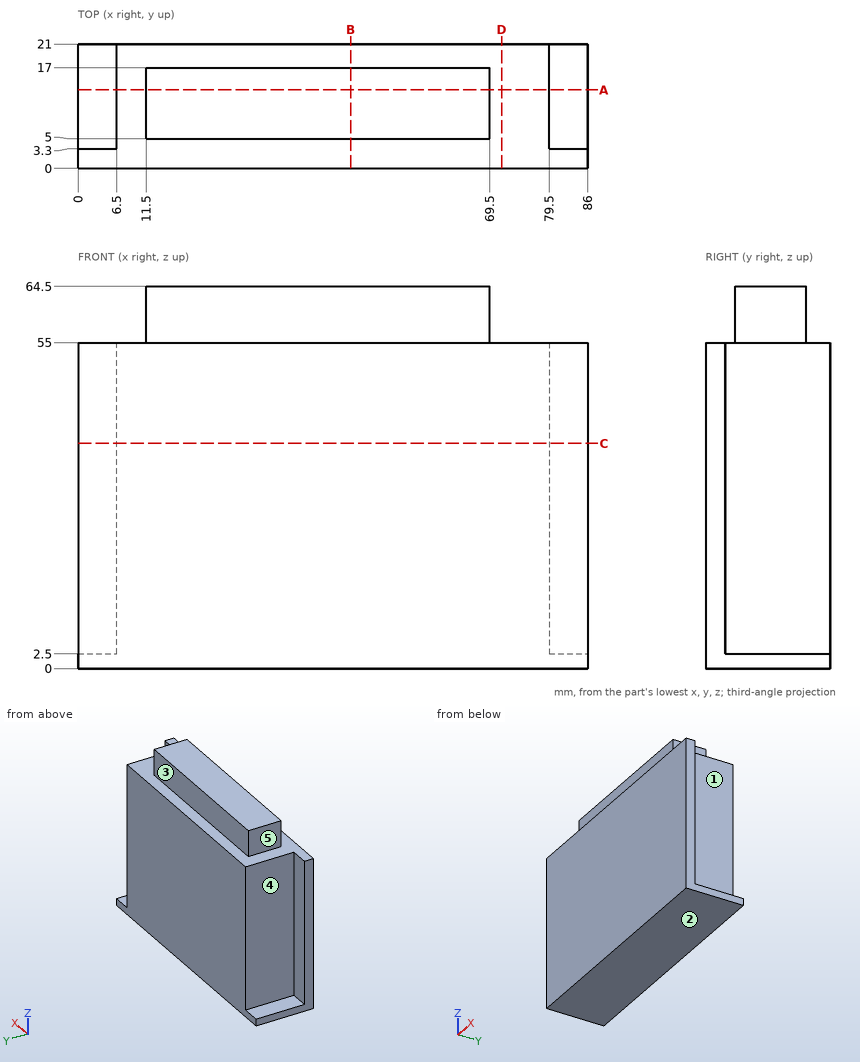
The figure shows three views and two pictorial views of one solid part (mm, origin at its lowest corner). Answer the questions. A direction names the side the tool comes from. Round coordinates to 2 decimals unless told otherwise and drop trailing zeros. Write each loop counter-clockwise with the first axis right and the second up, starting at its lowest first coordinate (ties: lowest second). Pieces come first, ordered by that corner, then holes. Notation, with made-up numbers: (-7.5, -12) - (48.5, -12) arc R20 cw to (48.5, 14) - close; hole circle Ø9 at (56, 20.25). An arc over 180 degrees is marked (long way). Use one line per item in the form item = value. Start each with the question number.
Item 1: A cutting plane is placed at D-D (x = 71.5). Write down the section's boundary in (y, z), plus the area to 4 significant figures.
Item 2: A cutting plane is placed at A-A (y = 13.25). Write down the section's boundary in (x, z), plus the area to 3 significant figures.
Item 3: A cutting plane is placed at B-B (x = 46). Write down the section's boundary in (y, z).
Item 4: A cutting plane is placed at C-C (z = 38). Write down the section's boundary in (x, y).
Item 5: Flat-ended cylindrical pins translate along their axes: pin 1 Ø5 at (y, z) = (9.5, 61.5) entering from -X; pin 2 Ø2 at (x, z) = (4.5, 32) entering from +Y; pin 3 Ø5.5 at (y, z) = (8, 37.5) entering from -X. Find the tip coordinate at first contact, or state that the pin passes through.
Item 6: Find the intervals of material crossed by line 1 (X direction, y = 8, z = 19.5); line 2 (Z direction, x = 29.5, y = 3); line 3 (Z direction, x = 5.5, y = 16.25), in increasing order. Write a range as [from, to].
Item 7: A tool of negligible diameter and unlimited length cuts with its end or side. For the marked faces 1, 2, 3, 4 and 5, from which of +Z, -Z, +X, -X, +Y, -Y can it reach the whole face along a straight path? Write none if from no direction.
The answers:
q1.outline = (0, 0) - (21, 0) - (21, 55) - (0, 55) - close
q1.area = 1,155 mm^2
q2.outline = (0, 0) - (86, 0) - (86, 2.5) - (79.5, 2.5) - (79.5, 55) - (69.5, 55) - (69.5, 64.5) - (11.5, 64.5) - (11.5, 55) - (6.5, 55) - (6.5, 2.5) - (0, 2.5) - close
q2.area = 4,600 mm^2
q3.outline = (0, 0) - (21, 0) - (21, 55) - (17, 55) - (17, 64.5) - (5, 64.5) - (5, 55) - (0, 55) - close
q4.outline = (0, 0) - (86, 0) - (86, 3.3) - (79.5, 3.3) - (79.5, 21) - (6.5, 21) - (6.5, 3.3) - (0, 3.3) - close
q5.pin_1 = 11.5
q5.pin_2 = 3.3
q5.pin_3 = 6.5
q6.line_1 = [6.5, 79.5]
q6.line_2 = [0, 55]
q6.line_3 = [0, 2.5]
q7.face_1 = +Z, +X, +Y
q7.face_2 = -Z, +X, -X, +Y, -Y
q7.face_3 = +Z, +X, -X, +Y
q7.face_4 = +Z, -X, +Y
q7.face_5 = +Z, -X, +Y, -Y
